Geometry: see drawing. Coordinates: mm, zero at the bounding-box minimum. Round coordinates to 2 decimals unless told otherwise and drop trailing zeros. Loops run counter-clockwise (first coordinate to the right, second up) from the corner with the lowest first, then second, coordinate; pieces in that order, holes last. Notation, with made-up numbers: (-3.5, 77) - (4.5, 77) arc R26 cw to (4.5, 96) - close; hole circle Ø8 at (54, 55). An arc over 180 degrees is marked (long way). Return JSON: item names as keys, results as strings. Group by question number.
1. First-contact query: pin 1 Ø10.5 at (x, y) = (14, 23) entering from +Z; pin 2 Ø3 at (y, z) = (36.5, 16) entering from -X; pin 3 Ø5 at (x, y) = (21.5, 24.5) entering from +Z; pin 4 Ø12 at (x, y) = (35, 18.5) entering from -Z. Flat tips, straight axial feed; report the tip coordinate or a pass-through.
2. Section C-C on z = 3.25. Return loops of the section in (x, y), and give its area (3 significant figures).
3. Material intervals for probe 1 along Y at (x, z) = (22.5, 16.5); probe 2 along Y at (x, z) = (22, 6); probe 3 along Y at (x, z) = (22.5, 25.25), sorted ascending.
4. Section D-D on z = 17. Return loops of the section in (x, y), and give its area (3 significant figures).
5. Draft query along Z for the marked faces 1, 2 and 3. Return one class per face: +Z half, -Z half, draft (parallel to the pull), parting line (faces both ways), or undercut.
6. Section A-A on y = 22.5. Return loops of the section in (x, z).
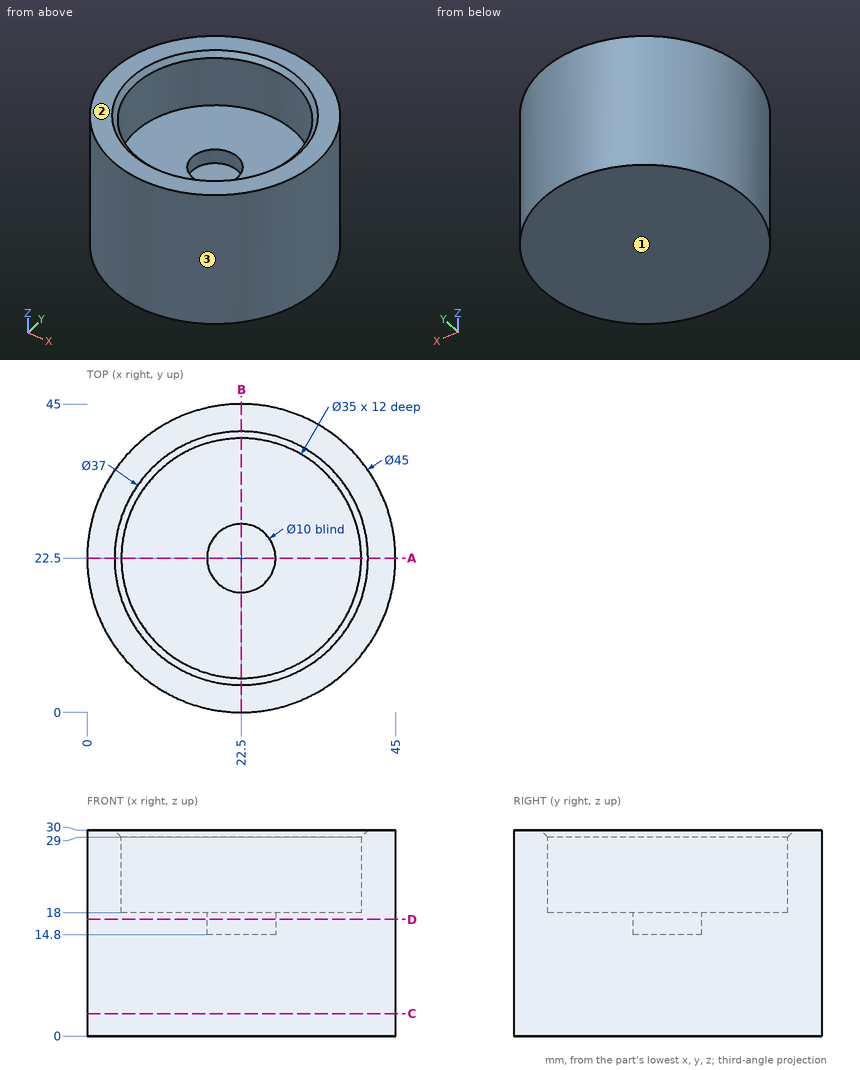
Taken from the geometry:
{
 "1": {"pin 1": "z = 18", "pin 2": "x = 3.79", "pin 3": "z = 14.8", "pin 4": "z = 0"},
 "2": {"outline": "circle Ø45 at (22.5, 22.5)", "area": "1,590 mm2"},
 "3": {"probe 1": "0 to 17.5, 27.5 to 45", "probe 2": "0.01 to 44.99", "probe 3": "0 to 5, 40 to 45"},
 "4": {"outline": "circle Ø45 at (22.5, 22.5); hole circle Ø10 at (22.5, 22.5)", "area": "1,510 mm2"},
 "5": {"face 1": "-Z half", "face 2": "+Z half", "face 3": "draft"},
 "6": {"outline": "(0, 0) - (45, 0) - (45, 30) - (41, 30) - (40, 29) - (40, 18) - (27.5, 18) - (27.5, 14.8) - (17.5, 14.8) - (17.5, 18) - (5, 18) - (5, 29) - (4, 30) - (0, 30) - close"}
}
